Can you work these out from the model? Positions are in its coordinate system, mm. Face numbers are marked on the shaded views. Give positions to 0.01 mm unless a question says otherwise; leave off trailing zeros. Loops run counter-clockwise (first coordinate to the right, second up) from the corner with the lowest first, then second, coordinate; pieces in that order, holes last.
from build123d import *

# Parameters (mm, degrees)
P_IDAT_VYSUNUT_M25_DEPTH      = 3
P_IDAT_VYSUNUT_M26_DEPTH      = 9.5
P_IDAT_VYSUNUT_M26_DEPTH_BACK = 3
SKICA1_21_W                   = 108.885125168
SKICA1_21_H                   = 128.6
P_IDAT_VYSUNUT_M28_DEPTH      = 6.8
SKICA1_24_R                   = 1.6
P_IDAT_VYSUNUT_M29_DEPTH      = 4.5
LINPOLE3_COUNT                = 2
LINPOLE3_PITCH                = 92
LINPOLE3_COUNT_DIR2           = 2
LINPOLE3_PITCH_DIR2           = 92
P_IDAT_VYSUNUT_M30_DEPTH      = 9.5
SKICA1_26_R                   = 1.6
P_IDAT_VYSUNUT_M31_DEPTH      = 7.2
LINPOLE4_COUNT                = 2
LINPOLE4_PITCH                = 92
LINPOLE4_COUNT_DIR2           = 2
LINPOLE4_PITCH_DIR2           = 113.2
SKICA8_W                      = 86.538297386
SKICA8_H                      = 86.538297386
P_IDAT_VYSUNUT_M32_DEPTH      = 5.5
ZAOBLIT4_R                    = 4
SKICA9_W                      = 22
SKICA9_H                      = 2.7
ODEBRAT_VYSUNUT_M1_DEPTH      = 10


with BuildPart() as part:
    # Skica1 → P_idat vysunut_m25 (new body)
    with BuildSketch(Plane(origin=(0, 0, 0), x_dir=(1, 0, 0), z_dir=(0, 1, 0))):
        Polygon((-51.442562584, -61.3), (51.442562584, -61.3), (51.442562584, 61.3), (-43.170983681, 61.3), (-43.228718708, 61.4), (-48.771281292, 61.4), (-48.829016319, 61.3), (-51.442562584, 61.3), (-51.442562584, 56.773205081), (-51.542562584, 56.6), (-51.442562584, 56.426794919), (-51.442562584, 46.173205081), (-51.542562584, 46), (-51.442562584, 45.826794919), align=None)
    extrude(amount=-P_IDAT_VYSUNUT_M25_DEPTH)

    # Skica1_21 → P_idat vysunut_m26 (add, two sides: drawn at the far end of the back side and taken through both)
    # profile 1 of 4: a face of its own
    with BuildSketch(Plane(origin=(0, 0, 0), x_dir=(1, 0, 0), z_dir=(0, 1, 0)).offset(-P_IDAT_VYSUNUT_M26_DEPTH_BACK)):
        Rectangle(SKICA1_21_W, SKICA1_21_H)
        Polygon((-51.442562584, -61.3), (-51.442562584, 45.826794919), (-51.542562584, 46), (-51.442562584, 46.173205081), (-51.442562584, 56.426794919), (-51.542562584, 56.6), (-51.442562584, 56.773205081), (-51.442562584, 61.3), (-48.829016319, 61.3), (-48.771281292, 61.4), (-43.228718708, 61.4), (-43.170983681, 61.3), (51.442562584, 61.3), (51.442562584, -61.3), align=None, mode=Mode.SUBTRACT)
    # profile 2 of 4: a face of its own
    with BuildSketch(Plane(origin=(0, 0, 0), x_dir=(1, 0, 0), z_dir=(0, 1, 0)).offset(-P_IDAT_VYSUNUT_M26_DEPTH_BACK)):
        Polygon((-51.542562584, 46), (-51.442562584, 45.826794919), (-51.442562584, 46.173205081), align=None)
    # profile 3 of 4: a face of its own
    with BuildSketch(Plane(origin=(0, 0, 0), x_dir=(1, 0, 0), z_dir=(0, 1, 0)).offset(-P_IDAT_VYSUNUT_M26_DEPTH_BACK)):
        Polygon((-51.542562584, 56.6), (-51.442562584, 56.426794919), (-51.442562584, 56.773205081), align=None)
    # profile 4 of 4: a face of its own
    with BuildSketch(Plane(origin=(0, 0, 0), x_dir=(1, 0, 0), z_dir=(0, 1, 0)).offset(-P_IDAT_VYSUNUT_M26_DEPTH_BACK)):
        Polygon((-48.829016319, 61.3), (-43.170983681, 61.3), (-43.228718708, 61.4), (-48.771281292, 61.4), align=None)
    extrude(amount=P_IDAT_VYSUNUT_M26_DEPTH + P_IDAT_VYSUNUT_M26_DEPTH_BACK)

    # Skica1_23 → P_idat vysunut_m28 (add)
    # profile 1 of 2: a face of its own
    with BuildSketch(Plane(origin=(0, 0, 0), x_dir=(1, 0, 0), z_dir=(0, 1, 0))):
        Polygon((-51.442562584, 45.826794919), (-48.771281292, 41.2), (-43.228718708, 41.2), (-40.457437416, 46), (-43.228718708, 50.8), (-48.771281292, 50.8), (-51.442562584, 46.173205081), align=None)
        Polygon((-44.383419246, 43.2), (-47.616580754, 43.2), (-49.233161507, 46), (-47.616580754, 48.8), (-44.383419246, 48.8), (-42.766838493, 46), align=None, mode=Mode.SUBTRACT)
    # profile 2 of 2: a face of its own
    with BuildSketch(Plane(origin=(0, 0, 0), x_dir=(1, 0, 0), z_dir=(0, 1, 0))):
        Polygon((-51.542562584, 46), (-51.442562584, 45.826794919), (-51.442562584, 46.173205081), align=None)
    p_idat_vysunut_m28 = extrude(amount=P_IDAT_VYSUNUT_M28_DEPTH)

    # Skica1_24 → P_idat vysunut_m29 (add)
    with BuildSketch(Plane(origin=(0, 0, 0), x_dir=(1, 0, 0), z_dir=(0, 1, 0))):
        Polygon((-49.233161507, 46), (-47.616580754, 43.2), (-44.383419246, 43.2), (-42.766838493, 46), (-44.383419246, 48.8), (-47.616580754, 48.8), align=None)
        with Locations(Location((-46, 46, 0), (0, 0, 270))):
            Circle(SKICA1_24_R, mode=Mode.SUBTRACT)
    p_idat_vysunut_m29 = extrude(amount=P_IDAT_VYSUNUT_M29_DEPTH)

    # LinPole3: P_idat vysunut_m28, P_idat vysunut_m29 2 × 2
    with Locations(*[(i * LINPOLE3_PITCH, 0, j * LINPOLE3_PITCH_DIR2) for i in range(LINPOLE3_COUNT) for j in range(LINPOLE3_COUNT_DIR2) if (i, j) != (0, 0)]):
        add(p_idat_vysunut_m28)
        add(p_idat_vysunut_m29)

    # Skica1_25 → P_idat vysunut_m30 (add)
    # profile 1 of 3: a face of its own
    with BuildSketch(Plane(origin=(0, 0, 0), x_dir=(1, 0, 0), z_dir=(0, 1, 0))):
        Polygon((-51.442562584, 56.773205081), (-51.442562584, 56.426794919), (-48.771281292, 51.8), (-43.228718708, 51.8), (-40.457437416, 56.6), (-43.170983681, 61.3), (-48.829016319, 61.3), align=None)
        Polygon((-43.2, 54.983419246), (-46, 53.366838493), (-48.8, 54.983419246), (-48.8, 58.216580754), (-46, 59.833161507), (-43.2, 58.216580754), align=None, mode=Mode.SUBTRACT)
    # profile 2 of 3: a face of its own
    with BuildSketch(Plane(origin=(0, 0, 0), x_dir=(1, 0, 0), z_dir=(0, 1, 0))):
        Polygon((-48.829016319, 61.3), (-43.170983681, 61.3), (-43.228718708, 61.4), (-48.771281292, 61.4), align=None)
    # profile 3 of 3: a face of its own
    with BuildSketch(Plane(origin=(0, 0, 0), x_dir=(1, 0, 0), z_dir=(0, 1, 0))):
        Polygon((-51.542562584, 56.6), (-51.442562584, 56.426794919), (-51.442562584, 56.773205081), align=None)
    p_idat_vysunut_m30 = extrude(amount=P_IDAT_VYSUNUT_M30_DEPTH)

    # Skica1_26 → P_idat vysunut_m31 (add)
    with BuildSketch(Plane(origin=(0, 0, 0), x_dir=(1, 0, 0), z_dir=(0, 1, 0))):
        Polygon((-48.8, 58.216580754), (-48.8, 54.983419246), (-46, 53.366838493), (-43.2, 54.983419246), (-43.2, 58.216580754), (-46, 59.833161507), align=None)
        with Locations(Location((-46, 56.6, 0), (0, 0, 270))):
            Circle(SKICA1_26_R, mode=Mode.SUBTRACT)
    p_idat_vysunut_m31 = extrude(amount=P_IDAT_VYSUNUT_M31_DEPTH)

    # LinPole4: P_idat vysunut_m30, P_idat vysunut_m31 2 × 2
    with Locations(*[(i * LINPOLE4_PITCH, 0, j * LINPOLE4_PITCH_DIR2) for i in range(LINPOLE4_COUNT) for j in range(LINPOLE4_COUNT_DIR2) if (i, j) != (0, 0)]):
        add(p_idat_vysunut_m30)
        add(p_idat_vysunut_m31)

    # Skica8 → P_idat vysunut_m32 (add)
    with BuildSketch(Plane(origin=(0, 0, 0), x_dir=(1, 0, 0), z_dir=(0, 1, 0))):
        Rectangle(SKICA8_W, SKICA8_H)
    extrude(amount=P_IDAT_VYSUNUT_M32_DEPTH)

    # Zaoblit4
    zaoblit4_edges = [part.edges().sort_by_distance(p)[0] for p in [
        (-54.442562584, 3.25, 64.3),
        (54.442562584, 3.25, 64.3),
        (54.442562584, 3.25, -64.3),
        (-54.442562584, 3.25, -64.3),
    ]]
    fillet(zaoblit4_edges, radius=ZAOBLIT4_R)

    # Skica9 → Odebrat vysunut_m1 (cut)
    with BuildSketch(Plane.ZY.offset(54.442562584)):
        with Locations((-30.8, 8.15)):
            Rectangle(SKICA9_W, SKICA9_H)
    extrude(amount=-ODEBRAT_VYSUNUT_M1_DEPTH, mode=Mode.SUBTRACT)


solid = part.part
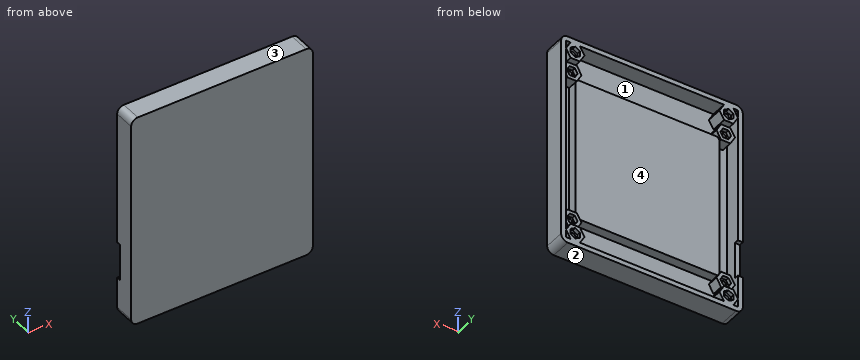
(1) Suppose I cut it at B-B on x = 4.5. List the corners of the cut face in (y, z) for me, plus the area to 3 significant figures.
Returned:
outline: (-3, -64.3) - (9.5, -64.3) - (9.5, -61.3) - (0, -61.3) - (0, -43.27) - (5.5, -43.27) - (5.5, 43.27) - (0, 43.27) - (0, 61.3) - (9.5, 61.3) - (9.5, 64.3) - (-3, 64.3) - close
area: 919 mm2
(2) Suppose I cut it at C-C on y = 3. Give the number of separate pieces and of enclosed holes in the cut face, plus the area to 3 significant figures.
Returned:
separate pieces: 1
enclosed holes: 16
area: 9,430 mm2
(3) Will these pins go through, and if not, where does the flat tip stop? P1, Ø2.5, axis at x = 46, z = 56.5, coming from the +Y side; P2, Ø3.5, axis at x = 46, z = 45.5, coming from the +Y side; P3, Ø0.8, axis at x = 50.5, z = -58.5, coming from the +Y side; P4, Ø5, axis at x = 46, z = -44, coming from the +Y side.
Returned:
P1: stops at y = 0
P2: stops at y = 4.5
P3: stops at y = 9.5
P4: stops at y = 6.8
(4) Thinking about a two-plate mould opening in Z: for the marked faces 1, 2, 3 and 4, which applies, pulls with the +Z half, pulls with the -Z half, needs draft (parallel to the pull), parting line crosses it, or undercut?
Returned:
face 1: undercut
face 2: pulls with the -Z half
face 3: pulls with the +Z half
face 4: undercut
(5) Please list where these lines run through material, in increasing order: probe 1 along X at (y, z) = (2, -56.6); probe 2 along Z at (x, y) = (11, 4.25); probe 3 along X at (y, z) = (3, 14).
Returned:
probe 1: x = -54.44 to -47.6, -44.4 to -40.46, 40.46 to 44.4, 47.6 to 54.44
probe 2: z = -64.3 to -61.3, -43.27 to 43.27, 61.3 to 64.3
probe 3: x = -54.44 to -51.44, -43.27 to 43.27, 51.44 to 54.44
(6) Suppose I cut it at A-A on z = -13.5. List the corners of the cut face in (x, y) for me.
Returned:
outline: (-54.44, -3) - (54.44, -3) - (54.44, 9.5) - (51.44, 9.5) - (51.44, 0) - (43.27, 0) - (43.27, 5.5) - (-43.27, 5.5) - (-43.27, 0) - (-51.44, 0) - (-51.44, 9.5) - (-54.44, 9.5) - close
